Input: part model. Units: mm. Frame: model coordinates. Face numbers are marked on the shaded views. A direction names the side the tool comes from. Round coordinates to 2 decimals unless told otherwise and drop trailing zeros. Loops run counter-clockwise (first coordinate to the right, second up) from the corner with the lowest first, then second, coordinate; pieces in that order, holes last. Notation, with made-up numbers: M 70.5,-25.75 L 102.5,-25.75 A19 ccw 102.5,-2.75 Z; hole C 28.25,42 d4. An arc over 180 degrees is marked long. Put each result on its own line as item: value. Start each with the question number.
1) Section A-A on x = 0. Output: boundary loops of the cut face in (y, z), plus the area to 3 significant figures.
2) Section B-B on z = -4.5. Output: boundary loops of the cut face in (x, y).
3) Reachability of the marked faces 1, 2 and 3 from +Z, -Z, +X, -X, +Y, -Y: full face, straight path, thin tool, end or side. Return the list, or none.
4) Draft query along X for the marked faces 4, 5 and 6. Return one class per face: +X half, -X half, draft (parallel to the pull), parting line (faces both ways), or undercut.
5) Section C-C on x = 38.1. Output: boundary loops of the cut face in (y, z), plus the area to 3 significant figures.
6) Pin query (flat end, axial travel): pin 1 (11.5 mm diameter, centred on x = 38.1, z = 0, fed in from +Y); pin 2 (1.5 mm diameter, centred on x = 13.5, z = 0, fed in from +Y); pin 3 (12.5 mm diameter, centred on x = -34.5, z = 4.5, fed in from +Y); pin 4 (6 mm diameter, centred on y = 30, z = 9, fed in from -X). Return the tip coordinate at first contact, or that it passes through.
7) Line query: probe 1 along X at (y, z) = (5.5, 0); probe 2 along Z at (x, y) = (-38.1, 2.75); probe 3 along Y at (x, z) = (0, 0.75). Output: solid intervals per line, ascending.
8) Section D-D on z = 2.25. Output: boundary loops of the cut face in (x, y), plus the area to 3 significant figures.
from build123d import *

# Parameters (mm, degrees)
SKETCH2_W           = 101.6
SKETCH2_H           = 25.4
BOSS_EXTRUDE1_DEPTH = 7.62
BOSS_EXTRUDE2_DEPTH = 12.7
SKETCH4_R           = 6.35635
CUT_EXTRUDE1_DEPTH  = 7.62
CUT_EXTRUDE2_REACH  = 27.4
SKETCH5_R           = 6.4135


with BuildPart() as part:
    # Sketch2 → Boss-Extrude1 (new body)
    with BuildSketch(Plane(origin=(0, 0, 0), x_dir=(1, 0, 0), z_dir=(0, 1, 0))):
        Rectangle(SKETCH2_W, SKETCH2_H)
    extrude(amount=BOSS_EXTRUDE1_DEPTH)

    # Sketch3 → Boss-Extrude2 (add, symmetric)
    with BuildSketch(Plane.XY):
        with BuildLine():
            ThreePointArc((25.4, 58.42), (0, 83.82), (-25.4, 58.42))
            Line((-25.4, 58.42), (25.4, 58.42))
        make_face()
        with BuildLine():
            Line((25.4, 58.42), (-25.4, 58.42))
            ThreePointArc((-25.4, 58.42), (0, 33.02), (25.4, 58.42))
        make_face()
        with BuildLine():
            Line((-25.4, 58.42), (-25.4, 7.62))
            Line((-25.4, 7.62), (25.4, 7.62))
            Line((25.4, 7.62), (25.4, 58.42))
            ThreePointArc((25.4, 58.42), (0, 33.02), (-25.4, 58.42))
        make_face()
    extrude(amount=BOSS_EXTRUDE2_DEPTH, both=True)

    # Sketch4 → Cut-Extrude1 (cut)
    with BuildSketch(Plane(origin=(0, 7.62, 0), x_dir=(1, 0, 0), z_dir=(0, 1, 0))):
        with Locations((38.1, 0)):
            Circle(SKETCH4_R)
    cut_extrude1 = extrude(amount=-CUT_EXTRUDE1_DEPTH, mode=Mode.SUBTRACT)

    # Mirror1: Cut-Extrude1 across plane
    add(cut_extrude1.mirror(Plane(origin=(0, 0, 0), x_dir=(0, 0, 1), z_dir=(1, 0, 0))), mode=Mode.SUBTRACT)

    # Sketch5 → Cut-Extrude2 (cut, up to next)
    with BuildSketch(Plane.XY.offset(12.7), mode=Mode.PRIVATE) as cut_extrude2_sk1:
        with Locations((0, 58.42)):
            Circle(SKETCH5_R)
    cut_extrude2_tool1 = extrude(cut_extrude2_sk1.sketch, amount=-CUT_EXTRUDE2_REACH, mode=Mode.PRIVATE) & part.part
    add(cut_extrude2_tool1.solids().sort_by_distance((0, 58.42, 12.7))[0], mode=Mode.SUBTRACT)


solid = part.part
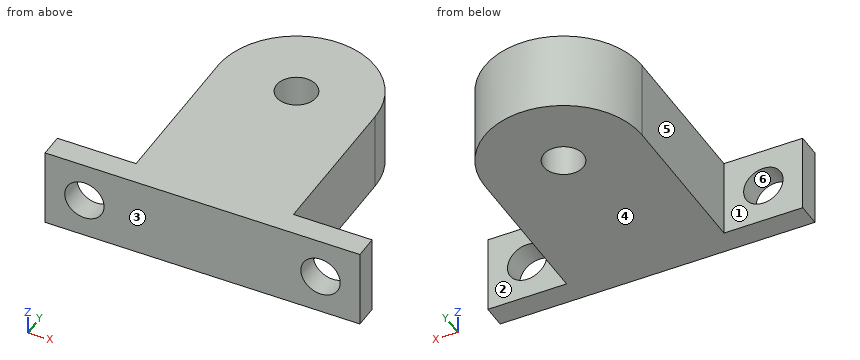
Geometry results:
1. outline: M 0,-12.7 L 52.01,-12.7 L 52.01,12.7 L 0,12.7 Z; M 64.83,-12.7 L 83.82,-12.7 L 83.82,12.7 L 64.83,12.7 Z
1. area: 1,800 mm²
2. outline: M -50.8,0 L -42.59,0 L -42.59,7.62 L -50.8,7.62 Z; M -33.61,0 L 33.61,0 L 33.61,7.62 L 25.4,7.62 L 25.4,58.42 A25.4 ccw -25.4,58.42 L -25.4,7.62 L -33.61,7.62 Z; M 42.59,0 L 50.8,0 L 50.8,7.62 L 42.59,7.62 Z; hole C 0,58.42 d12.83
3. face 1: +Z, -Z, -X, +Y
3. face 2: +Z, -Z, +X, +Y
3. face 3: +Z, -Z, +X, -X, -Y
4. face 4: draft
4. face 5: -X half
4. face 6: undercut
5. outline: M 0,-12.7 L 7.62,-12.7 L 7.62,-6.36 L 0,-6.36 Z; M 0,6.36 L 7.62,6.36 L 7.62,12.7 L 0,12.7 Z
5. area: 96.7 mm²
6. pin 1: passes through
6. pin 2: stops at y = 80.39
6. pin 3: stops at y = 7.62
6. pin 4: stops at x = -25.4
7. probe 1: x = -50.8 to -44.46, -31.74 to 31.74, 44.46 to 50.8
7. probe 2: z = -12.7 to -6.36, 6.36 to 12.7
7. probe 3: y = 0 to 52.01, 64.83 to 83.82
8. outline: M -50.8,0 L -44.04,0 L -44.04,7.62 L -50.8,7.62 Z; M -32.16,0 L 32.16,0 L 32.16,7.62 L 25.4,7.62 L 25.4,58.42 A25.4 ccw -25.4,58.42 L -25.4,7.62 L -32.16,7.62 Z; M 44.04,0 L 50.8,0 L 50.8,7.62 L 44.04,7.62 Z; hole C 0,58.42 d12.83
8. area: 4,060 mm²
